The drawing under review shows one solid part. Ordinate dimensions are in mm from its lowest x, y, z. Give positions to 0.01 mm unless a question says otherwise; leave off trailing zeros. Loops run counter-clockwise (first coordinate to the right, second up) from the corner with the lowest first, then second, coordinate; pieces in that order, holes last. Notation, with made-up numbers: M -39.75,58.25 L -23.75,58.25 A23 cw -23.75,70.25 Z; hole C -21,38 d6. An arc over 180 degrees is marked long. One line per item, written item: value. Start each with the question number.
Q1. For pin 1 (8 mm diameter, centred on x = 57, z = 43, fed in from +Y); pin 2 (1.5 mm diameter, centred on y = 22, z = 55.5, fed in from +X); pin 3 (10 mm diameter, centred on y = 75.5, z = 86.5, fed in from +X), all flat-tipped, find the tip position at first contact; note any pin that passes through.
Q2. To check wall thickness, follow line 1 along Y through (x, z) = (86.5, 61.5); line 2 along Z through (x, y) = (113, 89); line 3 along Y through (x, z) = (50, 16.5). State the ranges of each line that lie inside material, in increasing order. Write a range as from..to.
Q3. We need section C-C on z = 14.5. Write out the cut boundary in (x, y).
Q4. We need section D-D on z = 54. Write out the cut boundary in (x, y).
Q5. Mouldability with a two-part tool opening along X and no side actions: class the marked faces 1 and 2 as released by +X, released by -X, zero draft, split by the parting line, or undercut.
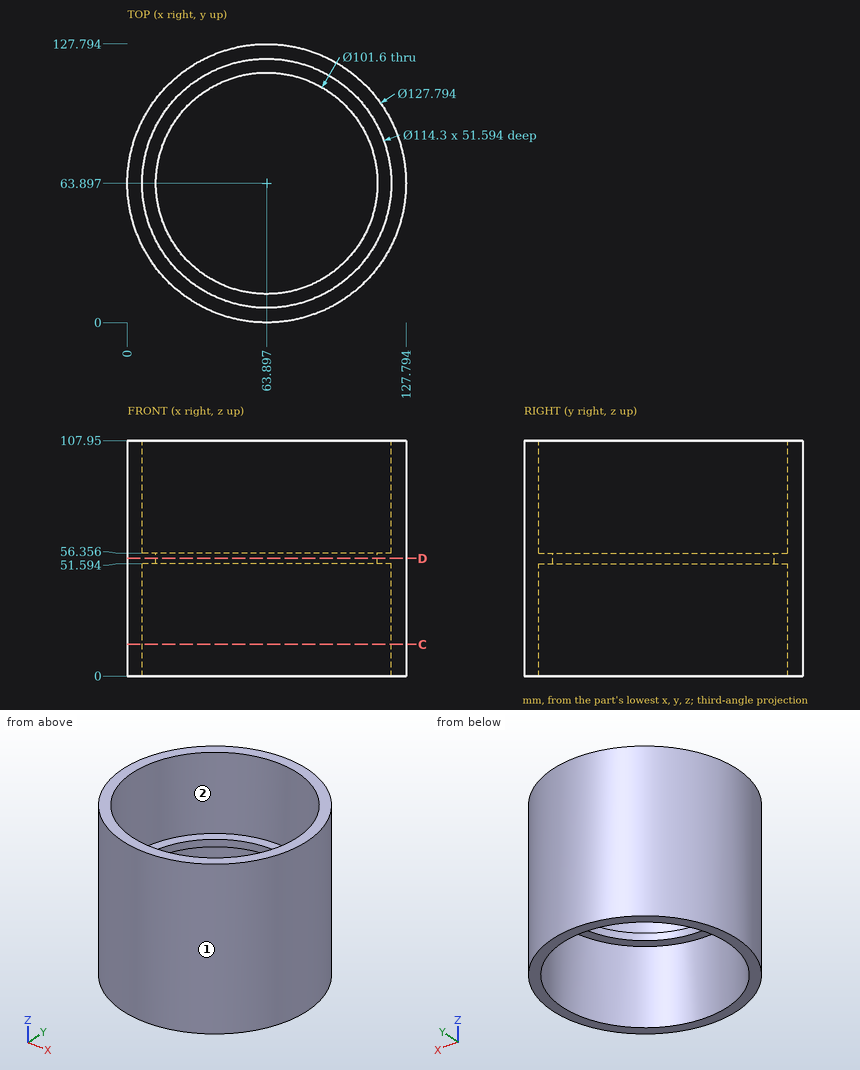
Solved:
1. pin 1: y = 127.73
1. pin 2: x = 112.78
1. pin 3: x = 127.45
2. line 1: 4.13..11.41, 116.39..123.66
2. line 2: 51.59..56.36
2. line 3: 1.53..8.46, 119.33..126.26
3. outline: C 63.9,63.9 d127.79; hole C 63.9,63.9 d114.3
4. outline: C 63.9,63.9 d127.79; hole C 63.9,63.9 d101.6
5. face 1: split by the parting line
5. face 2: undercut
